Can you work these out from the drawing? Everything is in mm from the part's minimum corner. Round coordinates to 2 decimals unless told otherwise and drop trailing zeros. Loops run counter-clockwise (first coordinate to the right, second up) from the corner with the lowest first, then second, coordinate; pieces in that order, holes last. Notation, with made-up numbers: (8.5, 86) -> (15.5, 86) arc R20 cw to (15.5, 113) -> close; hole circle Ø7 at (69, 83). An arc over 180 degrees is marked (long way). Answer as a JSON object with one key per item and string values.
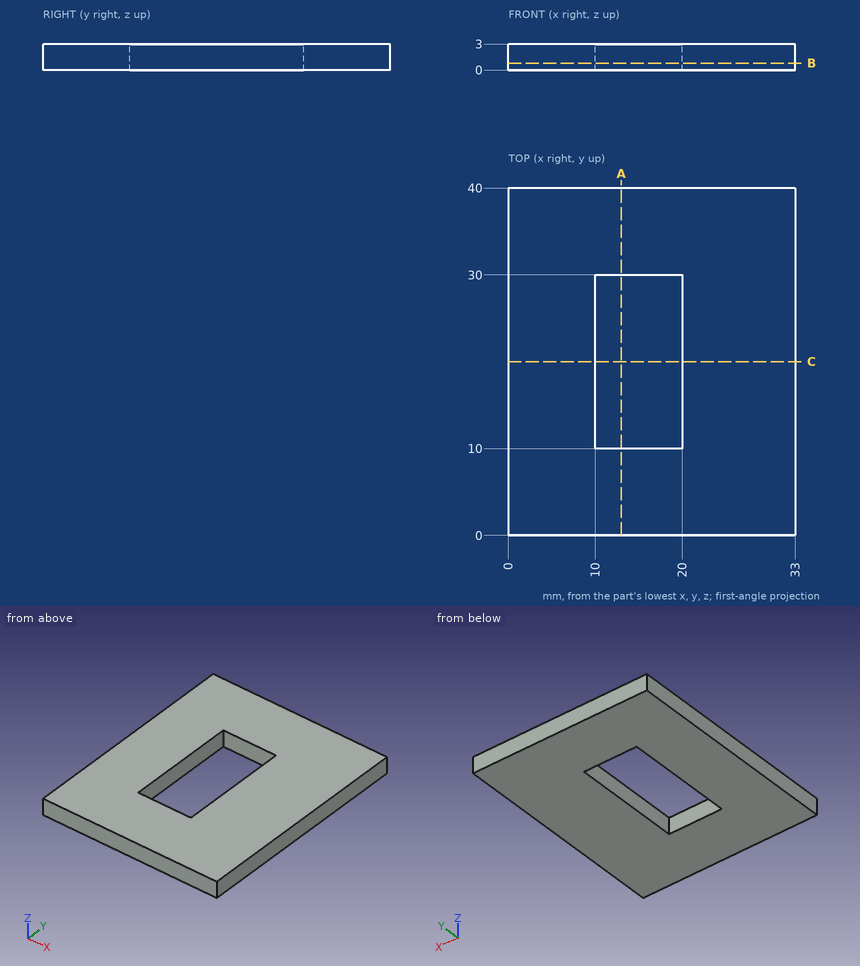
Q1. If I drill on L1, parallel to X at y = 20.5, z = 2.2; L2, parallel to Y at x = 17.5, z = 0.35, over which ranges is the centre line in solid material (lowest first)? Write a range as [from, to].
Determined:
{"L1": "[0, 10], [20, 33]", "L2": "[0, 10], [30, 40]"}
Q2. I want a section at C-C, the plane y = 20. Write out the boundary of the cut face in (x, z).
Determined:
{"outline": "(0, 0) -> (10, 0) -> (10, 3) -> (0, 3) -> close; (20, 0) -> (33, 0) -> (33, 3) -> (20, 3) -> close"}
Q3. I want a section at A-A, the plane x = 13. Write out the boundary of the cut face in (y, z), then the cut area to 3 significant figures.
Determined:
{"outline": "(0, 0) -> (10, 0) -> (10, 3) -> (0, 3) -> close; (30, 0) -> (40, 0) -> (40, 3) -> (30, 3) -> close", "area": "60.0 mm²"}
Q4. I want a section at B-B, the plane z = 0.8. Write out the boundary of the cut face in (x, y).
Determined:
{"outline": "(0, 0) -> (33, 0) -> (33, 40) -> (0, 40) -> close; hole (10, 10) -> (20, 10) -> (20, 30) -> (10, 30) -> close"}
